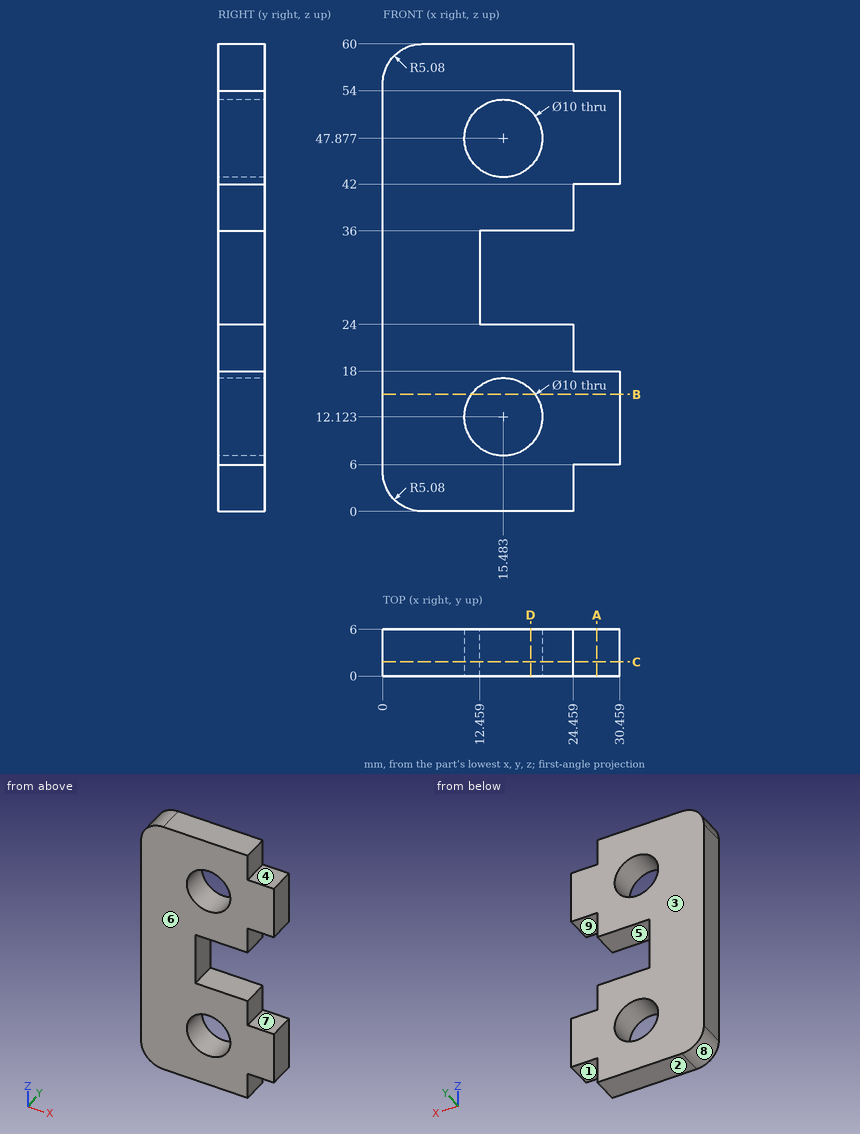
Job drawing, mm, ordinate dimensions from the low corner. One solid piece. A direction names the side the tool comes from. Give positions to 0.01 mm unless a question says otherwise; leave off trailing zeros. Write each loop counter-clockwise with the first axis right and the second up, starting at its lowest first coordinate (ties: lowest second). Pieces come first, ordered by that corner, then holes. Notation, with made-up numbers: M 31.25,30.5 L 85.25,30.5 A24 cw 85.25,51.5 Z; hole C 87,13.25 d11. An arc over 180 degrees is marked long. One line per item, written item: value. Start each with the question number.
Q1. Drop flat-ended pins along their axis: pin 1 Ø8 at (x, z) = (15.48, 12.12) entering from -Y; pin 2 Ø3 at (y, z) = (2.5, 57.5) entering from +X. Give the stop position or say it passes through.
Q2. Probe probe 1 along X at (y, z) = (4.55, 48) (1 decimal); probe 2 along Z at (x, y) = (11, 3.1) (1 decimal); probe 3 along Z at (x, y) = (14.5, 3.05) (1 decimal). List the from-to ranges inside material, lowest first. Write a range as [from, to].
Q3. 3-axis set-ups, long thin cutter, end or side, ignore diameter. For the marked faces 1, 2, 3, 4 and 5: which of +Z, -Z, +X, -X, +Y, -Y reach the whole face in a straight line?
Q4. Saw through at B-B, the plane z = 15. Write the cut outline in (x, y), plus the area to 3 significant figures.
Q5. Saw through at D-D, the plane x = 19. Write the cut outline in (y, z).
Q6. Saw through at A-A, the plane x = 27.5. Write the cut outline in (y, z).
Q7. Two-plate mould, pull along Z, no slides. Class the marked faces 6, 7, 8 and 9: +Z half, -Z half, draft (parallel to the pull), parting line (faces both ways), or undercut.
Q8. Saw through at C-C, the plane y = 1.8. Write the cut outline in (x, z).
Output values:
1. pin 1: passes through
1. pin 2: stops at x = 24.46
2. probe 1: x = [0, 10.5], [20.5, 30.5]
2. probe 2: z = [0, 9.9], [14.3, 45.7], [50.1, 60]
2. probe 3: z = [0, 7.2], [17, 24], [36, 43], [52.8, 60]
3. face 1: -Z, +X, +Y, -Y
3. face 2: -Z, +X, -X, +Y, -Y
3. face 3: +Z, -Z, +X, -X, +Y
3. face 4: +Z, +X, +Y, -Y
3. face 5: +X, +Y, -Y
4. outline: M 0,0 L 11.39,0 L 11.39,6 L 0,6 Z; M 19.57,0 L 30.46,0 L 30.46,6 L 19.57,6 Z
4. area: 134 mm²
5. outline: M 0,0 L 6,0 L 6,8.57 L 0,8.57 Z; M 0,15.68 L 6,15.68 L 6,24 L 0,24 Z; M 0,36 L 6,36 L 6,44.32 L 0,44.32 Z; M 0,51.43 L 6,51.43 L 6,60 L 0,60 Z
6. outline: M 0,6 L 6,6 L 6,18 L 0,18 Z; M 0,42 L 6,42 L 6,54 L 0,54 Z
7. face 6: draft
7. face 7: undercut
7. face 8: -Z half
7. face 9: undercut
8. outline: M 0,5.08 A5.08 ccw 5.08,0 L 24.46,0 L 24.46,6 L 30.46,6 L 30.46,18 L 24.46,18 L 24.46,24 L 12.46,24 L 12.46,36 L 24.46,36 L 24.46,42 L 30.46,42 L 30.46,54 L 24.46,54 L 24.46,60 L 5.08,60 A5.08 ccw 0,54.92 Z; hole C 15.48,12.12 d10; hole C 15.48,47.88 d10
